Could you check a few things on this model? Use its own coordinates, in mm. A direction names the side the tool comes from. Give positions to 0.01 mm unless a question says otherwise; leave off trailing zeros. Loops run counter-clockwise (first coordinate to the right, second up) from the corner with the lowest first, then second, coordinate; pieces in that order, holes last. Notation, with made-up numbers: (22.25, 14.25) - (62.25, 14.25) arc R26 ccw to (62.25, 39.25) - close; hole circle Ø10 at (72.25, 73). An arc over 180 degrees is marked (long way). Use CSV: the item, a comma, the result in double quotes.
from build123d import *

# Parameters (mm, degrees)
SALIENTE_EXTRUIR1_DEPTH = 9
CROQUIS2_R              = 3.5
CORTAR_EXTRUIR1_DEPTH   = 10
CROQUIS3_R              = 1.5
CORTAR_EXTRUIR2_DEPTH   = 10
SKETCH1_W               = 21.3
SKETCH1_H               = 7.15
BOSS_EXTRUDE1_DEPTH     = 2.8
SKETCH2_W               = 20
SKETCH2_H               = 6
CUT_EXTRUDE1_DEPTH      = 2.8


with BuildPart() as part:
    # Croquis1 → Saliente-Extruir1 (new body)
    with BuildSketch(Plane(origin=(0, 0, 0), x_dir=(1, 0, 0), z_dir=(0, 1, 0))):
        Polygon((0, 2.473088065), (2.473088065, 0), (32.526911935, 0), (35, 2.473088065), (35, 32.526911935), (32.526911935, 35), (2.473088065, 35), (0, 32.526911935), align=None)
    extrude(amount=SALIENTE_EXTRUIR1_DEPTH)

    # Croquis2 → Cortar-Extruir1 (cut, through all)
    with BuildSketch(Plane(origin=(0, 9, 0), x_dir=(1, 0, 0), z_dir=(0, 1, 0))):
        with Locations((17.5, 17.5)):
            Circle(CROQUIS2_R)
    extrude(amount=-CORTAR_EXTRUIR1_DEPTH, mode=Mode.SUBTRACT)

    # Croquis3 → Cortar-Extruir2 (cut, through all)
    with BuildSketch(Plane(origin=(0, 9, 0), x_dir=(1, 0, 0), z_dir=(0, 1, 0))):
        with Locations((4.5, 30.5)):
            Circle(CROQUIS3_R)
        with Locations((30.5, 30.5)):
            Circle(CROQUIS3_R)
        with Locations((30.5, 4.5)):
            Circle(CROQUIS3_R)
        with Locations((4.5, 4.5)):
            Circle(CROQUIS3_R)
    extrude(amount=-CORTAR_EXTRUIR2_DEPTH, mode=Mode.SUBTRACT)

    # Sketch1 → Boss-Extrude1 (add)
    with BuildSketch(Plane.ZY):
        with Locations((-17.5, 3.575)):
            Rectangle(SKETCH1_W, SKETCH1_H)
    extrude(amount=BOSS_EXTRUDE1_DEPTH)

    # Sketch2 → Cut-Extrude1 (cut)
    with BuildSketch(Plane.ZY.offset(2.8)):
        with Locations((-17.5, 3.575)):
            Rectangle(SKETCH2_W, SKETCH2_H)
    extrude(amount=-CUT_EXTRUDE1_DEPTH, mode=Mode.SUBTRACT)


solid = part.part
1) Suppose I cut it at C-C (y = 3). Please give me the cut outline in (x, z), plus the area to 3 significant figures.
Answer below:
outline,"(-2.8, -28.15) - (0, -28.15) - (0, -32.53) - (2.47, -35) - (32.53, -35) - (35, -32.53) - (35, -2.47) - (32.53, 0) - (2.47, 0) - (0, -2.47) - (0, -6.85) - (-2.8, -6.85) - (-2.8, -7.5) - (0, -7.5) - (0, -27.5) - (-2.8, -27.5) - close; hole circle Ø3 at (4.5, -30.5); hole circle Ø3 at (4.5, -4.5); hole circle Ø7 at (17.5, -17.5); hole circle Ø3 at (30.5, -30.5); hole circle Ø3 at (30.5, -4.5)"
area,"1,150 mm2"
2) I'm going to push flat-ended pins straight in: P1, Ø2.5, axis at x = 30.5, z = -30.5, coming from the -Y side; P2, Ø0.8, axis at x = -1.5, z = -13, coming from the +Y side; P3, Ø10, axis at x = 14, z = -14.5, coming from the -Y side; P4, Ø1, axis at y = 6, z = -20, coming from the -X side. Where does each tip first touch, or does it pass through?
Answer below:
P1,"passes through"
P2,"stops at y = 7.15"
P3,"stops at y = 0"
P4,"stops at x = 0"
3) We'd pull the mould along X, two halves only. Please class faces 1 (the cylindrical face through (5.886, 4.563, -3.925)), 2 (the flat face through (1.254, 4.437, -33.781)), 3 (the flat face through (18, 4, -35)): +X half, -X half, draft (parallel to the pull), parting line (faces both ways), or undercut.
Answer below:
face 1,"undercut"
face 2,"-X half"
face 3,"draft"
4) Suppose I cut it at B-B (x = 30.5). Please give me the cut outline in (y, z), plus the area to 3 significant figures.
Answer below:
outline,"(0, -35) - (9, -35) - (9, -32) - (0, -32) - close; (0, -29) - (9, -29) - (9, -6) - (0, -6) - close; (0, -3) - (9, -3) - (9, 0) - (0, 0) - close"
area,"261 mm2"
5) Which directions (+Z, -Z, +X, -X, +Y, -Y) give clear straight access to the entire face, cutting with the end or side of a thin tool? Please do faces 4 (the flat face through (-1, 0.575, -18)), 5 (the flat face through (33.746, 4.437, -1.219)), 6 (the flat face through (-1, 4, -6.85)), 7 (the flat face through (-1, 7.15, -18)), 8 (the flat face through (-1, 4, -28.15)).
Answer below:
face 4,"-X"
face 5,"+Z, +X, +Y, -Y"
face 6,"+Z, -X, +Y, -Y"
face 7,"+Z, -Z, -X, +Y"
face 8,"-Z, -X, +Y, -Y"
6) Suppose I cut it at D-D (z = -30.5). Please give me the cut outline in (x, y), plus the area to 3 significant figures.
Answer below:
outline,"(0, 0) - (3, 0) - (3, 9) - (0, 9) - close; (6, 0) - (29, 0) - (29, 9) - (6, 9) - close; (32, 0) - (35, 0) - (35, 9) - (32, 9) - close"
area,"261 mm2"
7) Suppose I cut it at A-A (z = -17.5). Please give me the cut outline in (x, y) (3 decimals), plus the area to 3 significant figures.
Answer below:
outline,"(-2.8, 0) - (14, 0) - (14, 9) - (0, 9) - (0, 7.15) - (-2.8, 7.15) - (-2.8, 6.575) - (0, 6.575) - (0, 0.575) - (-2.8, 0.575) - close; (21, 0) - (35, 0) - (35, 9) - (21, 9) - close"
area,"255 mm2"
8) I need wall thicknesses on line 1 along Z through (x, y) = (30.5, 4.5); line 2 along X through (y, z) = (4.5, -4.5); line 3 along Z through (x, y) = (17.5, 5). Which ranges of each line are inside material? Lowest first, please.
Answer below:
line 1,"z = -35 to -32, -29 to -6, -3 to 0"
line 2,"x = 0 to 3, 6 to 29, 32 to 35"
line 3,"z = -35 to -21, -14 to 0"
